```python
from build123d import *

# Parameters (mm, degrees)
F1_DEPTH = 25.4
F2_W     = 6.35
F2_H     = 12.7
F3_DEPTH = 25.4
F5_DEPTH = 12.7


with BuildPart() as f1:
    # F0 (on Right) → F1 (new body)
    with BuildSketch(Plane.YZ):
        Polygon((-25.4, 0), (0, 0), (0, 25.4), (-12.7, 25.4), (-25.4, 12.7), align=None)
    extrude(amount=F1_DEPTH)

    # F2 (on face) → F3 (join)
    with BuildSketch(Plane(origin=(0, 0, 0), x_dir=(0, -1, 0), z_dir=(-1, 0, 0))):
        with Locations((3.175, 6.35)):
            Rectangle(F2_W, F2_H)
    extrude(amount=F3_DEPTH)

    # F4 (on face) → F5 (join)
    with BuildSketch(Plane(origin=(-25.4, 0, 0), x_dir=(0, -1, 0), z_dir=(-1, 0, 0))):
        Polygon((6.35, 0), (25.4, 0), (13.477535, 12.7), (6.35, 12.7), align=None)
    extrude(amount=-F5_DEPTH)


solid = f1.part
```
Check sheet for the modelled part. Datum: model origin and axes. Units: mm. A direction names the side the tool comes from. Coordinates: 2 decimals unless noted, no trailing zeros. Order: outer loops, then holes, each group sorted by start corner. A loop starts at its lowest first (then second) coordinate and runs counter-clockwise, first axis right, second up. Notation, with made-up numbers: M -10.75,79 L 9.25,79 A27 ccw 9.25,102 Z; hole C -15,-24.5 d3. An arc over 180 degrees is marked long. Write each question's results on one line, items separated by ' | '. Start each with the question number.
1. Cross-section at D-D on y = -20.75. Record the cut outline in (x, z), and give its area (3 significant figures).
2. Material ranges on probe 1 along X at (y, z) = (-15, 9); probe 2 along X at (y, z) = (-21.25, 12); probe 3 along Z at (x, y) = (-21.5, -5), recorded low to high.
3. Cross-section at C-C on x = 1. Record the cut outline in (y, z), and give its area (3 significant figures).
4. Go/stop test with flat-tipped pins: P1, Ø6, axis at y = -16.5, z = 22.5, coming from the -X side; P2, Ø6.5, axis at x = -9, z = 6, coming from the -Y side; P3, Ø11, axis at x = -11.5, y = -8.5, coming from the +Z side. Record where each tip stops, or that it passes through.
5. Mould release check, pull along X, two halves, no side actions. Record for faces 1 (the face through (25.4, -13, 13)), 2 (the face through (0, -13, 13)), 3 (the face through (-12.7, -14, 5)), 4 (the face through (13, -25.4, 6)): +X half, -X half, draft (parallel to the pull), parting line (faces both ways), or undercut.
6. Cross-section at A-A on y = -7.5. Record the cut outline in (x, z).
7. Cross-section at B-B on z = 15.75. Record the cut outline in (x, y), and give its area (3 significant figures).
8. Access from +Z, -Z, +X, -X, +Y, -Y to the whole of each face (thin tool, end or side, straight path). Record for faces 5 (the face through (-6, -6.35, 6)), 6 (the face through (-19.139, -19.522, 6.261)), 7 (the face through (-16, -5, 12.7)).
Checks:
1) outline: M -25.4,0 L -12.7,0 L -12.7,4.95 L -25.4,4.95 Z; M 0,0 L 25.4,0 L 25.4,17.35 L 0,17.35 Z | area: 504 mm²
2) probe 1: x = -25.4 to -12.7, 0 to 25.4 | probe 2: x = 0 to 25.4 | probe 3: z = 0 to 12.7
3) outline: M -25.4,0 L 0,0 L 0,25.4 L -12.7,25.4 L -25.4,12.7 Z | area: 565 mm²
4) P1: stops at x = 0 | P2: stops at y = -6.35 | P3: stops at z = 12.7
5) face 1: +X half | face 2: undercut | face 3: undercut | face 4: draft
6) outline: M -25.4,0 L -12.7,0 L -12.7,12.7 L -25.4,12.7 Z; M 0,0 L 25.4,0 L 25.4,25.4 L 0,25.4 Z
7) outline: M 0,-22.35 L 25.4,-22.35 L 25.4,0 L 0,0 Z | area: 568 mm²
8) face 5: +Z, -Z, -Y | face 6: +Z, -X, -Y | face 7: +Z, -X, +Y, -Y
